Source: CAD feature listing. Evaluate the final solid. Frame: model axes, mm. Face numbers are marked on the shaded views. Give positions to 0.01 mm unless a question says otherwise; leave off trailing zeros. Loops run counter-clockwise (first coordinate to the right, second up) from the corner with the lowest first, then second, coordinate; pieces in that order, holes last. Notation, with made-up numbers: M -23,18 L 27,18 A23 ccw 27,38 Z; hole C 46,45.5 d4. An arc over 180 degrees is marked long. Put each result on its own line as item: value. Start each with the question number.
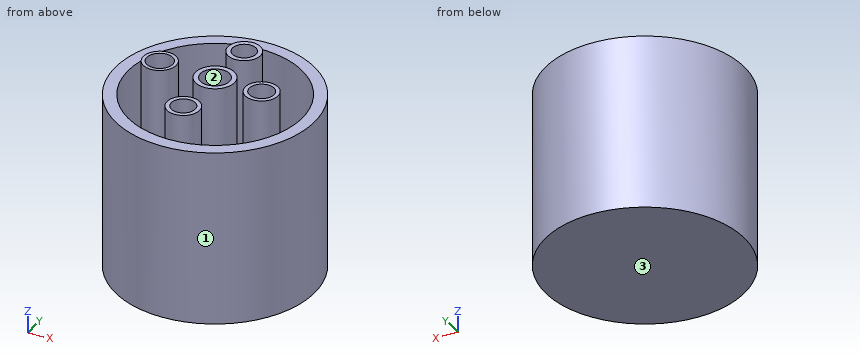
```python
from build123d import *

# Parameters (mm, degrees)
F0_R     = 56.334368
F0_R_2   = 49.169238
F1_DEPTH = 100
F3_DEPTH = 25
F4_DEPTH = 10
F5_R     = 11.028269
F5_R_2   = 8.205737
F5_R_3   = 9.231192
F5_R_4   = 6.622097
F5_R_5   = 9.284198
F5_R_6   = 6.989631
F5_R_7   = 9.315085
F5_R_8   = 7.337153
F5_R_9   = 9.189609
F5_R_10  = 6.786331
F6_DEPTH = 100


with BuildPart() as f1:
    # F0 (on Top) → F1 (new body)
    with BuildSketch(Plane.XY):
        Circle(F0_R)
        with Locations((0, 0.154715)):
            Circle(F0_R_2, mode=Mode.SUBTRACT)
    extrude(amount=F1_DEPTH)

    # F0 (on Top) → F3 (join)
    with BuildSketch(Plane.XY):
        Circle(F0_R)
        with Locations((0, 0.154715)):
            Circle(F0_R_2, mode=Mode.SUBTRACT)
    extrude(amount=F3_DEPTH)

    # F0 (on Top) → F4 (join)
    with BuildSketch(Plane.XY):
        with Locations((0, 0.154715)):
            Circle(F0_R_2)
    extrude(amount=F4_DEPTH)

    # F5 (on face) → F6 (join)
    with BuildSketch(Plane.XY.offset(10)):
        Circle(F5_R)
        Circle(F5_R_2, mode=Mode.SUBTRACT)
        with Locations((0, 29.241161)):
            Circle(F5_R_3)
        with Locations((0, 29.241161)):
            Circle(F5_R_4, mode=Mode.SUBTRACT)
        with Locations((26.920432, 0)):
            Circle(F5_R_5)
        with Locations((26.920432, 0)):
            Circle(F5_R_6, mode=Mode.SUBTRACT)
        with Locations((-31.871319, 0)):
            Circle(F5_R_7)
        with Locations((-31.871319, 0)):
            Circle(F5_R_8, mode=Mode.SUBTRACT)
        with Locations((0, -31.716604)):
            Circle(F5_R_9)
        with Locations((0, -31.716604)):
            Circle(F5_R_10, mode=Mode.SUBTRACT)
    extrude(amount=F6_DEPTH)


solid = f1.part
```
1. Section D-D, the plane x = 15. Output: boundary loops of the cut face in (y, z), plus the area to 3 significant figures.
2. Ray query, line 1 (Y direction, x = -33.5, z = 69.5); line 2 (Y direction, x = 25, z = 68); line 3 (Z direction, x = 41, y = -12). Return the intervals inside material, ascending.
3. Pull-direction query (X, two-part tool) for the marked faces 1, 2 and 3; classes: released by +X, released by -X, zero draft, split by the parting line, or undercut.
4. Section A-A, the plane z = 95.5. State how many separate pieces and enclosed holes the cut face has, plus the area to 3 significant figures.
5. Contact query for flat-ended pins moving along their axis: pin 1 (1 mm diameter, centred on x = 38.5, y = 2, fed in from +Z); pin 2 (10 mm diameter, centred on y = -40.5, z = 68, fed in from +X); pin 3 (6 mm diameter, centred on y = -14.5, z = 67, fed in from +X). Output: stop coordinate, or through.
Results found:
1. outline: M -54.3,0 L 54.3,0 L 54.3,100 L 46.98,100 L 46.98,10 L -46.67,10 L -46.67,100 L -54.3,100 Z
1. area: 2,430 mm²
2. line 1: -45.29 to -35.84, -9.17 to -7.15, 7.15 to 9.17, 36.15 to 45.29
2. line 2: -50.48 to -42.18, -9.08 to -6.72, 6.72 to 9.08, 42.49 to 50.48
2. line 3: 0 to 10
3. face 1: split by the parting line
3. face 2: undercut
3. face 3: zero draft
4. separate pieces: 6
4. enclosed holes: 6
4. area: 3,020 mm²
5. pin 1: z = 10
5. pin 2: x = 43.74
5. pin 3: x = 55.15
